Could you check a few things on this model? Use its own coordinates, in mm. A direction names the side the tool comes from. Give positions to 0.01 mm unless a question says otherwise; leave off trailing zeros. Order: outer loops, then holes, each group sorted by start corner. A loop starts at its lowest first (then second) coordinate and runs counter-clockwise, first axis right, second up. Notation, with made-up numbers: (75, -17.5) - (90, -17.5) arc R17 cw to (90, 10.5) - close; hole circle Ø9 at (30.25, -8). An arc over 180 degrees is marked (long way). One line per question, with ' | ' between items. Start each with the question number.
1. For P1, Ø3.5, axis at x = 8.5, y = -27.5, coming from the -Z side; P2, Ø1.5, axis at x = 0.5, y = -18, coming from the -Z side; P3, Ø3, axis at x = 5, z = 18, coming from the -Y side; P4, Ø10, axis at x = -3.5, z = 11, coming from the +Y side, each with a flat end and sliding along its axis, tell me the tip position at first contact or that it passes through.
2. If we mould it in two halves opening along X, with no side actions, what happens to faces 1 (the cylindrical face through (-1.526, -24.342, -24.845)), 2 (the flat face through (-6.219, 19, -15)), 3 (the flat face through (4, -27, -10))? For each: released by +X, released by -X, zero draft, split by the parting line, or undercut.
3. Imagine slicing it at D-D (x = -11). Please give me the cut outline in (y, z) (3 decimals).
4. I need wall thicknesses on probe 1 along Y at (x, z) = (-5, -23) (3 decimals); probe 2 along Y at (x, z) = (1.5, -11.5) (3 decimals); probe 3 along Y at (x, z) = (11.75, -11.5) (3 decimals). Which ranges of each line are inside material? Lowest first, please. Write a range as from..to.
5. Which directions (+Z, -Z, +X, -X, +Y, -Y) give clear straight access to the entire face, cutting with the end or side of a thin tool? Please do faces 4 (the flat face through (0, -9.075, -20)), 5 (the flat face through (5.281, -27, -7)), 6 (the flat face through (9.797, -27, -7)), 7 (the flat face through (-12, 19, -5)), 8 (the flat face through (0, -29.075, -13)).
6. Imagine slicing it at B-B (y = -22). Please give me the cut outline in (x, z), and give its area (3 significant figures).
7. Imagine slicing it at C-C (z = -20). Give the number of separate pieces and of enclosed holes in the cut face, and give its area (3 significant figures).
8. Imagine slicing it at A-A (z = -12.5). Please give me the cut outline in (x, y) (3 decimals).
```python
from build123d import *

# Parameters (mm, degrees)
SKETCH4_W                = 12.46
SKETCH4_H                = 17.25
BOSS_EXTRUDE3_DEPTH      = 6
SKETCH8_R                = 12.546781182
SKETCH8_R_2              = 11.15
BOSS_EXTRUDE6_DEPTH      = 7.3
BOSS_EXTRUDE6_DEPTH_BACK = 17.25
BOSS_EXTRUDE4_DEPTH      = 17.25
SKETCH6_R                = 0.5
CUT_EXTRUDE1_DEPTH       = 15
CHAMFER1_SIZE            = 0.5
CHAMFER1_SIZE2           = 0.866025404
SKETCH10_W               = 12.46
SKETCH10_H               = 23.7
CUT_EXTRUDE3_DEPTH       = 17.25
CUT_EXTRUDE4_REACH       = 38.097
SKETCH11_W               = 5
SKETCH11_H               = 3
BOSS_EXTRUDE7_DEPTH      = 7.3
BOSS_EXTRUDE9_DEPTH      = 10
SKETCH20_R               = 11.15
SKETCH20_R_2             = 7.15
BOSS_EXTRUDE11_DEPTH     = 7.3
SKETCH21_R               = 10.15
SKETCH21_R_2             = 7.15
CUT_EXTRUDE7_DEPTH       = 1.3
BOSS_EXTRUDE10_DEPTH     = 25.093562
SKETCH18_W               = 20
SKETCH18_H               = 12.438292938
CUT_EXTRUDE5_DEPTH       = 2
SKETCH19_R               = 1.25
CUT_EXTRUDE6_DEPTH       = 53.75
CUT_EXTRUDE6_DEPTH_BACK  = 3
FILLET1_R                = 10
SKETCH22_R               = 5.8
BOSS_EXTRUDE12_DEPTH     = 20
FILLET2_R                = 2
SKETCH23_R               = 5.930854157
SKETCH23_R_2             = 5.08
CUT_EXTRUDE8_DEPTH       = 11.6
SKETCH24_R               = 6.5
BOSS_EXTRUDE13_DEPTH     = 2
SKETCH25_R               = 1.25
BOSS_EXTRUDE14_DEPTH     = 2
SKETCH26_W               = 5
SKETCH26_H               = 3
BOSS_EXTRUDE15_DEPTH     = 5
SKETCH27_W               = 27.233314403
SKETCH27_H               = 38.605371191
CUT_EXTRUDE9_DEPTH       = 51.35
BOSS_EXTRUDE16_DEPTH     = 54.75
CUT_EXTRUDE10_DEPTH      = 13.546781182
CUT_EXTRUDE10_DEPTH_BACK = 13.546781182
CUT_EXTRUDE11_DEPTH      = 36


with BuildPart() as part:
    # Sketch4 → Boss-Extrude3 (new body)
    with BuildSketch(Plane.XY):
        with Locations((0, -1.35)):
            Rectangle(SKETCH4_W, SKETCH4_H)
    extrude(amount=BOSS_EXTRUDE3_DEPTH)



with BuildPart() as body_2:
    # Sketch8 → Boss-Extrude6 (new body, two sides)
    with BuildSketch(Plane(origin=(0, -9.975, 0), x_dir=(-1, 0, 0), z_dir=(0, -1, 0))) as boss_extrude6_sk:
        with Locations((0, -23.55)):
            Circle(SKETCH8_R)
        with Locations((0, -23.55)):
            Circle(SKETCH8_R_2, mode=Mode.SUBTRACT)
    extrude(amount=BOSS_EXTRUDE6_DEPTH)
    extrude(boss_extrude6_sk.sketch, amount=-BOSS_EXTRUDE6_DEPTH_BACK)


with BuildPart() as part_1:
    add(part.part)

    add(body_2.part)  # Boss-Extrude4 merges body 2
    # Sketch5 → Boss-Extrude4 (add)
    with BuildSketch(Plane(origin=(0, 7.275, 0), x_dir=(1, 0, 0), z_dir=(0, 1, 0))):
        with BuildLine():
            Line((12.546781182, -23.55), (12.546781182, 0))
            Line((12.546781182, 0), (6.23, 0))
            Line((6.23, 0), (6.23, -29.7))
            Line((6.23, -29.7), (-6.23, -29.7))
            Line((-6.23, -29.7), (-6.23, 0))
            Line((-6.23, 0), (-12.546781182, 0))
            Line((-12.546781182, 0), (-12.546781182, -23.55))
            ThreePointArc((-12.546781182, -23.55), (0, -36.096781182), (12.546781182, -23.55))
        make_face()
    extrude(amount=-BOSS_EXTRUDE4_DEPTH)

    # Sketch6 → Cut-Extrude1 (cut)
    with BuildSketch(Plane(origin=(0, 7.275, 0), x_dir=(1, 0, 0), z_dir=(0, 1, 0))):
        with Locations((0, -3.6)):
            Circle(SKETCH6_R)
        with Locations((0, -32.1)):
            Circle(SKETCH6_R)
    extrude(amount=-CUT_EXTRUDE1_DEPTH, mode=Mode.SUBTRACT)

    # Chamfer1
    chamfer1_edges = [part_1.edges().sort_by_distance(p)[0] for p in [
        (-0.5, 7.275, 3.6),
        (-0.5, 7.275, 32.1),
    ]]
    chamfer1_side = [part_1.faces().sort_by_distance(p)[0] for p in [
        (0, 7.275, 35.657160381),
    ]]
    chamfer(chamfer1_edges, length=CHAMFER1_SIZE, length2=CHAMFER1_SIZE2, reference=chamfer1_side[0])

    # Sketch10 → Cut-Extrude3 (cut)
    with BuildSketch(Plane(origin=(0, 7.275, 0), x_dir=(1, 0, 0), z_dir=(0, 1, 0))):
        with Locations((0, -17.85)):
            Rectangle(SKETCH10_W, SKETCH10_H)
    extrude(amount=-CUT_EXTRUDE3_DEPTH, mode=Mode.SUBTRACT)

    # Sketch11 → Cut-Extrude4 (cut, up to next)
    with BuildSketch(Plane.XY.offset(36.096781182), mode=Mode.PRIVATE) as cut_extrude4_sk1:
        with Locations((0, -8.475)):
            Rectangle(SKETCH11_W, SKETCH11_H)
    cut_extrude4_tool1 = extrude(cut_extrude4_sk1.sketch, amount=-CUT_EXTRUDE4_REACH, mode=Mode.PRIVATE) & part_1.part
    add(cut_extrude4_tool1.solids().sort_by_distance((0, -8.475, 36.096781))[0], mode=Mode.SUBTRACT)

    # Sketch13 → Boss-Extrude7 (add)
    with BuildSketch(Plane.XZ.offset(17.275)):
        with BuildLine():
            Line((-12.546781182, 23.55), (-12.546781182, 0))
            Line((-12.546781182, 0), (12.546781182, 0))
            Line((12.546781182, 0), (12.546781182, 23.55))
            ThreePointArc((12.546781182, 23.55), (0, 11.003218818), (-12.546781182, 23.55))
        make_face()
    extrude(amount=-BOSS_EXTRUDE7_DEPTH)

    # Sketch15 → Boss-Extrude9 (add)
    with BuildSketch(Plane(origin=(0, 7.275, 0), x_dir=(1, 0, 0), z_dir=(0, 1, 0))):
        with BuildLine():
            Line((-12.546781182, 0), (12.546781182, 0))
            Line((12.546781182, 0), (12.546781182, -23.55))
            ThreePointArc((12.546781182, -23.55), (0, -36.096781182), (-12.546781182, -23.55))
            Line((-12.546781182, -23.55), (-12.546781182, 0))
        make_face()
        with BuildLine():
            Line((-6.23, -0.8), (6.23, -0.8))
            Line((6.23, -0.8), (6.23, -33.5))
            ThreePointArc((6.23, -33.5), (5.937106781, -34.207106781), (5.23, -34.5))
            Line((5.23, -34.5), (-5.23, -34.5))
            ThreePointArc((-5.23, -34.5), (-5.937106781, -34.207106781), (-6.23, -33.5))
            Line((-6.23, -33.5), (-6.23, -0.8))
        make_face(mode=Mode.SUBTRACT)
    extrude(amount=BOSS_EXTRUDE9_DEPTH)

    # Sketch20 → Boss-Extrude11 (add)
    with BuildSketch(Plane.XZ.offset(17.275)):
        with Locations((0, 23.55)):
            Circle(SKETCH20_R)
        with Locations((0, 23.55)):
            Circle(SKETCH20_R_2, mode=Mode.SUBTRACT)
    extrude(amount=-BOSS_EXTRUDE11_DEPTH)

    # Sketch21 → Cut-Extrude7 (cut)
    with BuildSketch(Plane.XZ.offset(17.275)):
        with Locations((0, 23.55)):
            Circle(SKETCH21_R)
        with Locations((0, 23.55)):
            Circle(SKETCH21_R_2, mode=Mode.SUBTRACT)
    extrude(amount=-CUT_EXTRUDE7_DEPTH, mode=Mode.SUBTRACT)

    # Sketch17 → Boss-Extrude10 (add)
    with BuildSketch(Plane(origin=(12.546781182, 4.728218818, 0), x_dir=(0, 1, 0), z_dir=(-1, 0, 0))):
        Polygon((16.946781182, 25), (16.946781182, 0), (-37.803218818, 0), (-37.803218818, 25), (-33.803218818, 25), (-33.803218818, 5), (12.946781182, 5), (12.946781182, 25), align=None)
    extrude(amount=BOSS_EXTRUDE10_DEPTH)

    # Sketch18 → Cut-Extrude5 (cut)
    with BuildSketch(Plane(origin=(0, 17.675, 0), x_dir=(0, 0, 1), z_dir=(0, -1, 0))):
        with Locations((-15, 0)):
            Rectangle(SKETCH18_W, SKETCH18_H)
    extrude(amount=-CUT_EXTRUDE5_DEPTH, mode=Mode.SUBTRACT)

    # Sketch19 → Cut-Extrude6 (cut, two sides)
    with BuildSketch(Plane(origin=(0, 19.675, 0), x_dir=(0, 0, 1), z_dir=(0, -1, 0))) as cut_extrude6_sk:
        with Locations((-20, 0)):
            Circle(SKETCH19_R)
    extrude(amount=CUT_EXTRUDE6_DEPTH, mode=Mode.SUBTRACT)
    extrude(cut_extrude6_sk.sketch, amount=-CUT_EXTRUDE6_DEPTH_BACK, mode=Mode.SUBTRACT)

    # Fillet1
    fillet1_edges = [part_1.edges().sort_by_distance(p)[0] for p in [
        (-12.546780818, 19.675, -25),
        (12.546781182, 19.675, -25),
        (12.546781182, -31.075, -25),
        (-12.546780818, -31.075, -25),
    ]]
    fillet(fillet1_edges, radius=FILLET1_R)

    # Sketch22 → Boss-Extrude12 (add)
    with BuildSketch(Plane(origin=(0, -29.075, 0), x_dir=(0, 0, -1), z_dir=(0, 1, 0))):
        with Locations((20, 0)):
            Circle(SKETCH22_R)
    extrude(amount=BOSS_EXTRUDE12_DEPTH)

    # Fillet2
    fillet2_edges = [part_1.edges().sort_by_distance(p)[0] for p in [
        (0, -9.075, -14.2),
    ]]
    fillet(fillet2_edges, radius=FILLET2_R)

    # Sketch23 → Cut-Extrude8 (cut)
    with BuildSketch(Plane(origin=(0, -29.075, 0), x_dir=(0, 0, -1), z_dir=(0, 1, 0))):
        with Locations((20, 0)):
            Circle(SKETCH23_R)
        with Locations((20, 0)):
            Circle(SKETCH23_R_2, mode=Mode.SUBTRACT)
    extrude(amount=CUT_EXTRUDE8_DEPTH, mode=Mode.SUBTRACT)

    # Sketch24 → Boss-Extrude13 (add)
    with BuildSketch(Plane(origin=(0, -17.475, 0), x_dir=(0, 0, 1), z_dir=(0, -1, 0))):
        with Locations((-20, 0)):
            Circle(SKETCH24_R)
    extrude(amount=BOSS_EXTRUDE13_DEPTH)

    # Sketch25 → Boss-Extrude14 (add)
    with BuildSketch(Plane(origin=(0, -33.075, 0), x_dir=(0, 0, 1), z_dir=(0, -1, 0))):
        with Locations((-20, 0)):
            Circle(SKETCH25_R)
    extrude(amount=-BOSS_EXTRUDE14_DEPTH)

    # Sketch26 → Boss-Extrude15 (add)
    with BuildSketch(Plane(origin=(0, -29.075, 0), x_dir=(0, 0, -1), z_dir=(0, 1, 0))):
        with Locations((7.5, -8.296781182)):
            Rectangle(SKETCH26_W, SKETCH26_H)
        with Locations((7.5, -3.780781182)):
            Rectangle(SKETCH26_W, SKETCH26_H)
    extrude(amount=BOSS_EXTRUDE15_DEPTH)

    # Sketch27 → Cut-Extrude9 (cut, through all)
    with BuildSketch(Plane(origin=(0, 17.275, 0), x_dir=(1, 0, 0), z_dir=(0, 1, 0))):
        with Locations((1.06987602, -19.302685596)):
            Rectangle(SKETCH27_W, SKETCH27_H)
    extrude(amount=-CUT_EXTRUDE9_DEPTH, mode=Mode.SUBTRACT)

    # Sketch28 → Boss-Extrude16 (add)
    with BuildSketch(Plane(origin=(0, 21.675, 0), x_dir=(1, 0, 0), z_dir=(0, 1, 0))):
        Polygon((12.546781182, 0), (0, -30), (-12.546781182, 0), align=None)
    extrude(amount=-BOSS_EXTRUDE16_DEPTH)

    # Sketch29 → Cut-Extrude10 (cut, two sides)
    with BuildSketch(Plane(origin=(0, 0, 0), x_dir=(0, 0, -1), z_dir=(1, 0, 0))) as cut_extrude10_sk:
        Polygon((0, 21.675), (-30, 21.675), (-30, 0), align=None)
        Polygon((0, -33.075), (-30, -33.075), (-30, -0.02), align=None)
    extrude(amount=CUT_EXTRUDE10_DEPTH, mode=Mode.SUBTRACT)
    extrude(cut_extrude10_sk.sketch, amount=-CUT_EXTRUDE10_DEPTH_BACK, mode=Mode.SUBTRACT)

    # Sketch30 → Cut-Extrude11 (cut, through all)
    with BuildSketch(Plane(origin=(0, 0, -5), x_dir=(-1, 0, 0), z_dir=(0, 0, -1))):
        Polygon((12.546781182, 21.675), (0, 0), (12.546781182, -29.075), align=None)
    extrude(amount=-CUT_EXTRUDE11_DEPTH, mode=Mode.SUBTRACT)


solid = part_1.part
```
Results found:
1) P1: stops at z = -23.55 | P2: stops at z = -26.5 | P3: stops at y = -14.89 | P4: stops at y = 17.34
2) face 1: split by the parting line | face 2: undercut | face 3: zero draft
3) outline: (-33.075, -20.343) - (-29.075, -20.343) - (-29.075, -5) - (-25.491, -5) - (-25.491, 3.698) - (-29, 3.698) - (-33.075, 0) - close; (17.675, -20.343) - (21.675, -20.343) - (21.675, 0) - (19.003, 3.698) - (19.003, -5) - (17.675, -5) - close
4) probe 1: y = -33.075..-29.075, -19.475..-17.475, 19.675..21.675 | probe 2: y = -33.075..-29.075, 19.675..21.675 | probe 3: y = -33.075..-29.075, 17.675..21.675
5) face 4: -Z, +X, -X | face 5: -Z | face 6: -Z, +X | face 7: +Z, -X | face 8: none
6) outline: (-9.49, -5) - (12.55, -5) - (12.55, 0) - (8.34, 10.05) - (-8.34, 10.05) - (-9.49, 7.3) - close; circle Ø10.16 at (0, -20) | area: 390 mm2
7) separate pieces: 3 | enclosed holes: 1 | area: 364 mm2
8) outline: (-12.547, -33.075) - (12.547, -33.075) - (12.547, -29.075) - (-12.547, -29.075) - close; (-12.547, 17.675) - (-6.219, 17.675) - (-6.219, 19.675) - (6.219, 19.675) - (6.219, 17.675) - (12.547, 17.675) - (12.547, 21.675) - (-12.547, 21.675) - close
